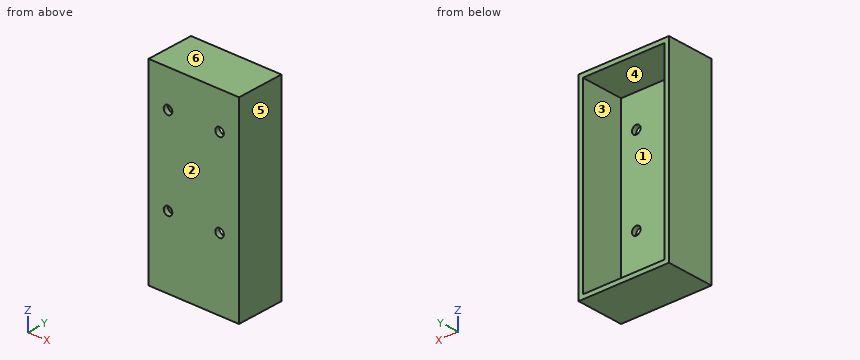
from build123d import *

# Parameters (mm, degrees)
SKETCH_1_W          = 42.1
SKETCH_1_H          = 89.8
EXTRUDE_1_DEPTH     = 22.2
SKETCH_2_W          = 38.1
SKETCH_2_H          = 85.8
CUT_EXTRUDE_1_DEPTH = 20
SKETCH_3_R          = 2
CUT_EXTRUDE_2_DEPTH = 54.47066953


with BuildPart() as part:
    # 스케치1 → 보스-돌출1 (new body)
    with BuildSketch(Plane(origin=(0, 0, 0), x_dir=(1, 0, 0), z_dir=(0, 1, 0))):
        Rectangle(SKETCH_1_W, SKETCH_1_H)
    extrude(amount=EXTRUDE_1_DEPTH)

    # 스케치2 → 컷-돌출1 (cut)
    with BuildSketch(Plane(origin=(0, 22.2, 0), x_dir=(1, 0, 0), z_dir=(0, 1, 0))):
        Rectangle(SKETCH_2_W, SKETCH_2_H)
    extrude(amount=-CUT_EXTRUDE_1_DEPTH, mode=Mode.SUBTRACT)

    # 스케치3 → 컷-돌출2 (cut, through all)
    with BuildSketch(Plane(origin=(0, 2.2, 0), x_dir=(1, 0, 0), z_dir=(0, 1, 0))):
        with Locations(Location((-12, -27.9, 0), (0, 0, 270))):
            Circle(SKETCH_3_R)
        with Locations(Location((-12, 12.1, 0), (0, 0, 270))):
            Circle(SKETCH_3_R)
        with Locations(Location((12, 12.1, 0), (0, 0, 270))):
            Circle(SKETCH_3_R)
        with Locations(Location((12, -27.9, 0), (0, 0, 270))):
            Circle(SKETCH_3_R)
    extrude(amount=-CUT_EXTRUDE_2_DEPTH, mode=Mode.SUBTRACT)


solid = part.part
Can you work these out from the model? Positions are in its coordinate system, mm. Face numbers are marked on the shaded views. A direction names the side the tool comes from. Give positions to 0.01 mm unless a question says otherwise; leave off trailing zeros. Order: outer loops, then holes, each group sorted by start corner. A loop starts at its lowest first (then second) coordinate and runs counter-clockwise, first axis right, second up. Notation, with made-up numbers: M 59,81.5 L 96,81.5 A24 cw 96,104.5 Z; hole C 79.25,32.25 d11. An arc over 180 degrees is marked long. Use a Markdown table: item, result. Add a question column.
Item 1: Suppose I cut it at B-B (x = 12). List the corners of the cut face in (y, z) for me.
Item 2: Will these pins go through, and if not, where does the flat tip stop? pin 1 (2.5 mm diameter, centred on x = 12, z = 27.9, fed in from +Y); pin 2 (5 mm diameter, centred on x = -7, z = 29, fed in from +Y).
Item 3: If I drill on L1, parallel to X at y = 1.4, z = 27.9; L2, parallel to X at y = 9.25, z = 3.5; L3, parallel to Z at x = -3.5, y = 8.75, over which ranges is the centre line in solid material (lowest first)? Write a range as [from, to].
Item 4: For the marked faces 1 and 2, which set-ups out of +Z, -Z, +X, -X, +Y, -Y let a thin tool reach every point of the face, with its end or its side?
Item 5: We'd pull the mould along X, two halves only. Please class the marked faces 3, 4, 5 and 6: +X half, -X half, draft (parallel to the pull), parting line (faces both ways), or undercut.
Item 6: Suppose I cut it at D-D (z = 20). List the corners of the cut face in (x, y) for me.
Item 7: Suppose I cut it at C-C (y = 4.25). List the corners of the cut face in (x, z) for me, then the cut area to 3 significant figures.
Item 8: Suppose I cut it at A-A (z = -12.1). List the corners of the cut face in (x, y) for me, then the cut area to 3 significant figures.
Answer sheet:
| question | item | result |
|---|---|---|
| 1 | outline | M 0,-44.9 L 22.2,-44.9 L 22.2,-42.9 L 2.2,-42.9 L 2.2,-14.1 L 0,-14.1 Z; M 0,-10.1 L 2.2,-10.1 L 2.2,25.9 L 0,25.9 Z; M 0,29.9 L 2.2,29.9 L 2.2,42.9 L 22.2,42.9 L 22.2,44.9 L 0,44.9 Z |
| 2 | pin 1 | passes through |
| 2 | pin 2 | stops at y = 2.2 |
| 3 | L1 | x = [-21.05, -14], [-10, 10], [14, 21.05] |
| 3 | L2 | x = [-21.05, -19.05], [19.05, 21.05] |
| 3 | L3 | z = [-44.9, -42.9], [42.9, 44.9] |
| 4 | face 1 | +Y |
| 4 | face 2 | +Z, -Z, +X, -X, -Y |
| 5 | face 3 | undercut |
| 5 | face 4 | undercut |
| 5 | face 5 | +X half |
| 5 | face 6 | draft |
| 6 | outline | M -21.05,0 L 21.05,0 L 21.05,22.2 L 19.05,22.2 L 19.05,2.2 L -19.05,2.2 L -19.05,22.2 L -21.05,22.2 Z |
| 7 | outline | M -21.05,-44.9 L 21.05,-44.9 L 21.05,44.9 L -21.05,44.9 Z; hole M -19.05,-42.9 L 19.05,-42.9 L 19.05,42.9 L -19.05,42.9 Z |
| 7 | area | 512 mm² |
| 8 | outline | M -21.05,0 L -14,0 L -14,2.2 L -19.05,2.2 L -19.05,22.2 L -21.05,22.2 Z; M -10,0 L 10,0 L 10,2.2 L -10,2.2 Z; M 14,0 L 21.05,0 L 21.05,22.2 L 19.05,22.2 L 19.05,2.2 L 14,2.2 Z |
| 8 | area | 155 mm² |
